Input: part model. Units: mm. Frame: model coordinates. Coordinates: 2 decimals unless noted, no trailing zeros. Order: outer loops, then holes, each group sorted by start corner. A loop starts at its lowest first (then second) coordinate and runs counter-clockwise, first axis right, second up. Notation, with made-up numbers: (-37.5, 58.5) -> (1.5, 58.5) arc R23 ccw to (1.5, 76.5) -> close; hole circle Ø8 at (61.25, 33.5). An arc over 180 degrees is marked (long way). One line per question, with ' | ' between items.
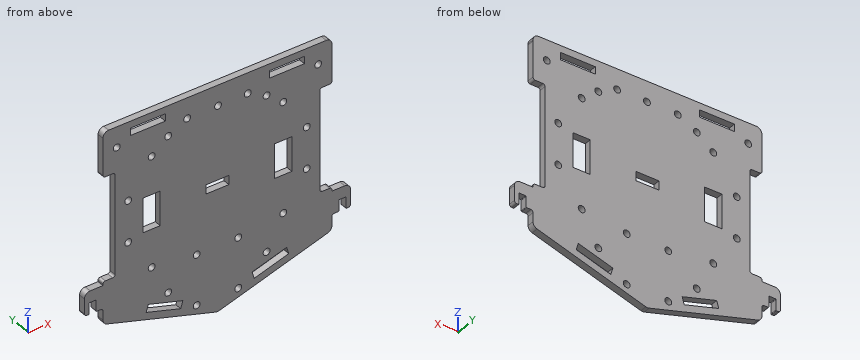
```python
from build123d import *

# Parameters (mm, degrees)
CROQUIS3_R              = 1.5
CROQUIS3_W              = 10
CROQUIS3_H              = 4
CROQUIS3_W_2            = 7.5
CROQUIS3_H_2            = 15
SALIENTE_EXTRUIR1_DEPTH = 3
CROQUIS4_R              = 1.5
CROQUIS4_W              = 14
CROQUIS4_H              = 45
CROQUIS4_W_2            = 15.2
CROQUIS4_H_2            = 3.2
CORTAR_EXTRUIR1_DEPTH   = 3
SALIENTE_EXTRUIR2_DEPTH = 3
REDONDEO1_R             = 1
REDONDEO2_R             = 0.25
CROQUIS9_R              = 1.5
CORTAR_EXTRUIR3_DEPTH   = 5


with BuildPart() as part:
    # Croquis3 → Saliente-Extruir1 (new body)
    with BuildSketch(Plane(origin=(0, 0, 0), x_dir=(1, 0, 0), z_dir=(0, 1, 0))):
        with BuildLine():
            Line((-50, -40), (50, -40))
            Line((50, -40), (50, 23.189923373))
            Line((50, 23.189923373), (55.6, 23.189923373))
            ThreePointArc((55.6, 23.189923373), (57.367766953, 23.92215642), (58.1, 25.689923373))
            Line((58.1, 25.689923373), (58.1, 33.189923373))
            Line((58.1, 33.189923373), (56.1, 33.189923373))
            Line((56.1, 33.189923373), (56.1, 28.189923373))
            Line((56.1, 28.189923373), (53, 28.189923373))
            Line((53, 28.189923373), (53, 33.189923373))
            Line((53, 33.189923373), (50, 33.189923373))
            Line((50, 33.189923373), (50, 38.139923373))
            ThreePointArc((50, 38.139923373), (49.505732321, 39.632249697), (48.218369714, 40.534489086))
            Line((48.218369714, 40.534489086), (0.718369714, 54.784489086))
            ThreePointArc((0.718369714, 54.784489086), (0, 54.889923373), (-0.718369714, 54.784489086))
            Line((-0.718369714, 54.784489086), (-48.218369714, 40.534489086))
            ThreePointArc((-48.218369714, 40.534489086), (-49.505732321, 39.632249697), (-50, 38.139923373))
            Line((-50, 38.139923373), (-50, 33.189923373))
            Line((-50, 33.189923373), (-53, 33.189923373))
            Line((-53, 33.189923373), (-53, 28.189923373))
            Line((-53, 28.189923373), (-56.1, 28.189923373))
            Line((-56.1, 28.189923373), (-56.1, 33.189923373))
            Line((-56.1, 33.189923373), (-58.1, 33.189923373))
            Line((-58.1, 33.189923373), (-58.1, 25.689923373))
            ThreePointArc((-58.1, 25.689923373), (-57.367766953, 23.92215642), (-55.6, 23.189923373))
            Line((-55.6, 23.189923373), (-50, 23.189923373))
            Line((-50, 23.189923373), (-50, -40))
        make_face()
        with Locations(Location((-21.533414662, 37.830612774, 0), (0, 0, 270))):
            Circle(CROQUIS3_R, mode=Mode.SUBTRACT)
        with Locations(Location((21.466585338, 37.830612774, 0), (0, 0, 270))):
            Circle(CROQUIS3_R, mode=Mode.SUBTRACT)
        with Locations(Location((21.466585338, -29.811737192, 0), (0, 0, 270))):
            Circle(CROQUIS3_R, mode=Mode.SUBTRACT)
        with Locations(Location((-21.533414662, -29.811737192, 0), (0, 0, 270))):
            Circle(CROQUIS3_R, mode=Mode.SUBTRACT)
        Rectangle(CROQUIS3_W, CROQUIS3_H, mode=Mode.SUBTRACT)
        with Locations((28.75, 0)):
            Rectangle(CROQUIS3_W_2, CROQUIS3_H_2, mode=Mode.SUBTRACT)
        with Locations((-28.75, 0)):
            Rectangle(CROQUIS3_W_2, CROQUIS3_H_2, mode=Mode.SUBTRACT)
        Polygon((-31.156326057, 42.52101023), (-16.056326057, 47.05101023), (-15.126326057, 43.95101023), (-30.226326057, 39.42101023), align=None, mode=Mode.SUBTRACT)
        Polygon((15.126326057, 43.95101023), (30.226326057, 39.42101023), (31.156326057, 42.52101023), (16.056326057, 47.05101023), align=None, mode=Mode.SUBTRACT)
    extrude(amount=SALIENTE_EXTRUIR1_DEPTH)

    # Croquis4 → Cortar-Extruir1 (cut, symmetric)
    with BuildSketch(Plane(origin=(0, 3, 0), x_dir=(1, 0, 0), z_dir=(0, 1, 0))):
        with Locations(Location((28.75, 24, 0), (0, 0, 270))):
            Circle(CROQUIS4_R)
        with Locations(Location((-28.75, 24, 0), (0, 0, 270))):
            Circle(CROQUIS4_R)
        with Locations(Location((28.75, -24, 0), (0, 0, 270))):
            Circle(CROQUIS4_R)
        with Locations(Location((-28.75, -24, 0), (0, 0, 270))):
            Circle(CROQUIS4_R)
        with Locations(Location((0.25, -34.055868596, 0), (0, 0, 270))):
            Circle(CROQUIS4_R)
        with Locations(Location((-13.25, -34.055868596, 0), (0, 0, 270))):
            Circle(CROQUIS4_R)
        with Locations(Location((13.25, -34.055868596, 0), (0, 0, 270))):
            Circle(CROQUIS4_R)
        with Locations(Location((-39, 9, 0), (0, 0, 270))):
            Circle(CROQUIS4_R)
        with Locations(Location((39, 9, 0), (0, 0, 270))):
            Circle(CROQUIS4_R)
        with Locations(Location((39, -9, 0), (0, 0, 270))):
            Circle(CROQUIS4_R)
        with Locations(Location((-39, -9, 0), (0, 0, 270))):
            Circle(CROQUIS4_R)
        with Locations(Location((-43.980956203, -34.055868596, 0), (0, 0, 270))):
            Circle(CROQUIS4_R)
        with Locations(Location((43.980956203, -34.055868596, 0), (0, 0, 270))):
            Circle(CROQUIS4_R)
        with Locations((51.75, -0.930038314)):
            Rectangle(CROQUIS4_W, CROQUIS4_H)
        with Locations((-51.75, -0.930038314)):
            Rectangle(CROQUIS4_W, CROQUIS4_H)
        with Locations((-30.4, -38.4)):
            Rectangle(CROQUIS4_W_2, CROQUIS4_H_2)
        with Locations((30.4, -38.4)):
            Rectangle(CROQUIS4_W_2, CROQUIS4_H_2)
    extrude(amount=CORTAR_EXTRUIR1_DEPTH, both=True, mode=Mode.SUBTRACT)

    # Croquis5 → Saliente-Extruir2 (add)
    with BuildSketch(Plane(origin=(0, 0, 0), x_dir=(1, 0, 0), z_dir=(0, 1, 0))):
        with BuildLine():
            Line((-50, -40), (49.999265674, -40))
            Line((49.999265674, -40), (49.999265674, -40.5))
            ThreePointArc((49.999265674, -40.5), (49.267032626, -42.267766953), (47.499265674, -43))
            Line((47.499265674, -43), (-47.5, -43))
            ThreePointArc((-47.5, -43), (-49.267766953, -42.267766953), (-50, -40.5))
            Line((-50, -40.5), (-50, -40))
        make_face()
    extrude(amount=SALIENTE_EXTRUIR2_DEPTH)

    # Redondeo1
    redondeo1_edges = [part.edges().sort_by_distance(p)[0] for p in [
        (-50, 1.5, -21.569961686),
        (-50, 1.5, 23.430038314),
        (50, 1.5, -21.569961686),
        (50, 1.5, 23.430038314),
        (-44.75, 1.5, -21.569961686),
        (-44.75, 1.5, 23.430038314),
        (44.75, 1.5, 23.430038314),
        (44.75, 1.5, -21.569961686),
        (-58.1, 1.5, -33.189923373),
        (-50, 1.5, -33.189923373),
        (50, 1.5, -33.189923373),
        (58.1, 1.5, -33.189923373),
    ]]
    fillet(redondeo1_edges, radius=REDONDEO1_R)

    # Redondeo2
    redondeo2_edges = [part.edges().sort_by_distance(p)[0] for p in [
        (-56.1, 1.5, -33.189923373),
        (-56.1, 1.5, -28.189923373),
        (-53, 1.5, -28.189923373),
        (-53, 1.5, -33.189923373),
        (53, 1.5, -33.189923373),
        (53, 1.5, -28.189923373),
        (56.1, 1.5, -28.189923373),
        (56.1, 1.5, -33.189923373),
    ]]
    fillet(redondeo2_edges, radius=REDONDEO2_R)

    # Croquis9 → Cortar-Extruir3 (cut, symmetric)
    with BuildSketch(Plane(origin=(0, 3, 0), x_dir=(1, 0, 0), z_dir=(0, 1, 0))):
        with Locations(Location((-9.075164729, 48.441511714, 0), (0, 0, 270))):
            Circle(CROQUIS9_R)
        with Locations(Location((-9.075164729, 26.572395433, 0), (0, 0, 270))):
            Circle(CROQUIS9_R)
        with Locations(Location((9.075164729, 26.572395433, 0), (0, 0, 270))):
            Circle(CROQUIS9_R)
        with Locations(Location((9.075164729, 48.441511714, 0), (0, 0, 270))):
            Circle(CROQUIS9_R)
    extrude(amount=CORTAR_EXTRUIR3_DEPTH, both=True, mode=Mode.SUBTRACT)


solid = part.part
```
1. Ray query, line 1 (X direction, y = 1.85, z = 37.5); line 2 (X direction, y = 2.15, z = 0); line 3 (Z direction, x = 40, y = 2.1). Return the intervals inside material, ascending. Write a range as [from, to].
Recorded:
line 1: x = [-50, -38], [-22.8, 22.8], [38, 50] | line 2: x = [-44.75, -32.5], [-25, -5], [5, 25], [32.5, 44.75] | line 3: z = [-43, -10.12], [-7.88, 7.88], [10.12, 43]
2. Pin query (flat end, axial travel): pin 1 Ø3 at (x, z) = (26.5, -6.5) entering from -Y; pin 2 Ø0.9 at (y, z) = (2, 39) entering from +X; pin 3 Ø1 at (x, y) = (20.5, 0.5) entering from -Z. Return the tip coordinate at first contact, or that it passes through.
Recorded:
pin 1: stops at y = 0 | pin 2: stops at x = 50 | pin 3: stops at z = -49
3. Cut plane B-B, the plane x = 13.25. Return loops of the section in (y, z) (3 decimals).
Recorded:
outline: (0, -51.025) -> (3, -51.025) -> (3, 32.556) -> (0, 32.556) -> close; (0, 35.556) -> (3, 35.556) -> (3, 43) -> (0, 43) -> close
4. Cut plane A-A, the plane z = 9. Return loops of the section in (x, y).
Recorded:
outline: (-44.75, 0) -> (-40.5, 0) -> (-40.5, 3) -> (-44.75, 3) -> close; (-37.5, 0) -> (37.5, 0) -> (37.5, 3) -> (-37.5, 3) -> close; (40.5, 0) -> (44.75, 0) -> (44.75, 3) -> (40.5, 3) -> close
5. Cut plane D-D, the plane y = 0.5. State how many separate pieces and enclosed holes the cut face has, and give its area (3 significant figures).
Recorded:
separate pieces: 1 | enclosed holes: 28 | area: 8,090 mm^2
6. Cut plane C-C, the plane x = -28.75. Return loops of the section in (y, z) (3 decimals), and give its area (3 significant figures).
Recorded:
outline: (0, -46.375) -> (3, -46.375) -> (3, -43.243) -> (0, -43.243) -> close; (0, -39.864) -> (3, -39.864) -> (3, -25.5) -> (0, -25.5) -> close; (0, -22.5) -> (3, -22.5) -> (3, -7.5) -> (0, -7.5) -> close; (0, 7.5) -> (3, 7.5) -> (3, 22.5) -> (0, 22.5) -> close; (0, 25.5) -> (3, 25.5) -> (3, 36.8) -> (0, 36.8) -> close; (0, 40) -> (3, 40) -> (3, 43) -> (0, 43) -> close | area: 185 mm^2
